```python
from build123d import *

# Parameters (mm, degrees)
SKETCH_1_W                         = 54
SKETCH_1_H                         = 25
SKETCH_1_R                         = 4
SKETCH_1_R_2                       = 1.5
SM_BASE_FLANGE_1_DEPTH             = 2
SM_EDGE_FLANGE_1_STRIP_W           = 10.4732
SM_EDGE_FLANGE_1_STRIP_H           = 2
SM_EDGE_FLANGE_1_STRIP_CUT_DEPTH   = 25
SM_EDGE_FLANGE_1_STRIP_2_W         = 10.4732
SM_EDGE_FLANGE_1_STRIP_2_H         = 2
SM_EDGE_FLANGE_1_STRIP_CUT_2_DEPTH = 25
SM_EDGE_FLANGE_1_DEPTH             = 25
SM_EDGE_FLANGE_1_BEND_DEPTH        = 25
SKETCH_12_R                        = 4
SKETCH_12_R_2                      = 1.5
CUT_EXTRUDE_1_DEPTH                = 72


# Sheet-metal steps are written as plain solids
with BuildPart() as part:
    # Sketch 1 → 基体-法兰1 (new body)
    with BuildSketch(Plane.XY):
        with Locations((27, -12.5)):
            Rectangle(SKETCH_1_W, SKETCH_1_H)
        with Locations((27, -12.5)):
            Circle(SKETCH_1_R, mode=Mode.SUBTRACT)
        with Locations((27, -5.5)):
            Circle(SKETCH_1_R_2, mode=Mode.SUBTRACT)
        with Locations((27, -19.5)):
            Circle(SKETCH_1_R_2, mode=Mode.SUBTRACT)
        with Locations((34, -12.5)):
            Circle(SKETCH_1_R_2, mode=Mode.SUBTRACT)
        with Locations((20, -12.5)):
            Circle(SKETCH_1_R_2, mode=Mode.SUBTRACT)
        with Locations((45.5, -12.5)):
            Circle(SKETCH_1_R_2, mode=Mode.SUBTRACT)
        with Locations((8.5, -12.5)):
            Circle(SKETCH_1_R_2, mode=Mode.SUBTRACT)
    extrude(amount=-SM_BASE_FLANGE_1_DEPTH)

    # 边线-法兰1 strip (across the edge) → 边线-法兰1 strip cut (cut)
    with BuildSketch(Plane(origin=(-1, 0, 0), x_dir=(1, 0, 0), z_dir=(0, -1, 0))):
        with Locations((-2.5, -1)):
            Rectangle(SM_EDGE_FLANGE_1_STRIP_W, SM_EDGE_FLANGE_1_STRIP_H)
    extrude(amount=SM_EDGE_FLANGE_1_STRIP_CUT_DEPTH, mode=Mode.SUBTRACT)

    # 边线-法兰1 strip 2 (across the edge) → 边线-法兰1 strip cut 2 (cut)
    with BuildSketch(Plane(origin=(55, -25, 0), x_dir=(-1, 0, 0), z_dir=(0, 1, 0))):
        with Locations((-2.5, -1)):
            Rectangle(SM_EDGE_FLANGE_1_STRIP_2_W, SM_EDGE_FLANGE_1_STRIP_2_H)
    extrude(amount=SM_EDGE_FLANGE_1_STRIP_CUT_2_DEPTH, mode=Mode.SUBTRACT)

    # 边线-法兰1 section (across the edge) → 边线-法兰1 (add)
    with BuildSketch(Plane(origin=(-1, 0, 0), x_dir=(1, 0, 0), z_dir=(0, -1, 0))):
        with BuildLine():
            Line((0, 0.7366), (0, 68))
            Line((0, 68), (2, 68))
            Line((2, 68), (2, 0.7366))
            ThreePointArc((2, 0.7366), (2.215745145, 0.215745145), (2.7366, 0))
            Line((2.7366, 0), (2.7366, -2))
            ThreePointArc((2.7366, -2), (0.801531583, -1.198468417), (0, 0.7366))
        make_face()
    extrude(amount=SM_EDGE_FLANGE_1_DEPTH)

    # 边线-法兰1 section 2 (across the edge) → 边线-法兰1 bend (add)
    with BuildSketch(Plane(origin=(55, -25, 0), x_dir=(-1, 0, 0), z_dir=(0, 1, 0))):
        with BuildLine():
            Line((0, 0.7366), (0, 68))
            Line((0, 68), (2, 68))
            Line((2, 68), (2, 0.7366))
            ThreePointArc((2, 0.7366), (2.215745145, 0.215745145), (2.7366, 0))
            Line((2.7366, 0), (2.7366, -2))
            ThreePointArc((2.7366, -2), (0.801531583, -1.198468417), (0, 0.7366))
        make_face()
    extrude(amount=SM_EDGE_FLANGE_1_BEND_DEPTH)

    # 草图12 → 切除-拉伸1 (cut)
    with BuildSketch(Plane(origin=(55, 0, 0), x_dir=(0, 0, -1), z_dir=(1, 0, 0))):
        with Locations(Location((-50, -12.5, 0), (0, 0, 180))):
            Circle(SKETCH_12_R)
        with Locations(Location((-57, -12.5, 0), (0, 0, 180))):
            Circle(SKETCH_12_R_2)
        with Locations(Location((-50, -5.5, 0), (0, 0, 180))):
            Circle(SKETCH_12_R_2)
        with Locations(Location((-43, -12.5, 0), (0, 0, 180))):
            Circle(SKETCH_12_R_2)
        with Locations(Location((-50, -19.5, 0), (0, 0, 180))):
            Circle(SKETCH_12_R_2)
        with Locations(Location((-31.5, -12.5, 0), (0, 0, 180))):
            Circle(SKETCH_12_R_2)
        with Locations(Location((-14.5, -12.5, 0), (0, 0, 180))):
            Circle(SKETCH_12_R_2)
        with BuildLine():
            Line((-49.5, -25), (-68, -25))
            Line((-68, -25), (-68, 0))
            Line((-68, 0), (-49.5, 0))
            ThreePointArc((-49.5, 0), (-62, -12.5), (-49.5, -25))
        make_face()
    extrude(amount=-CUT_EXTRUDE_1_DEPTH, mode=Mode.SUBTRACT)


solid = part.part
```
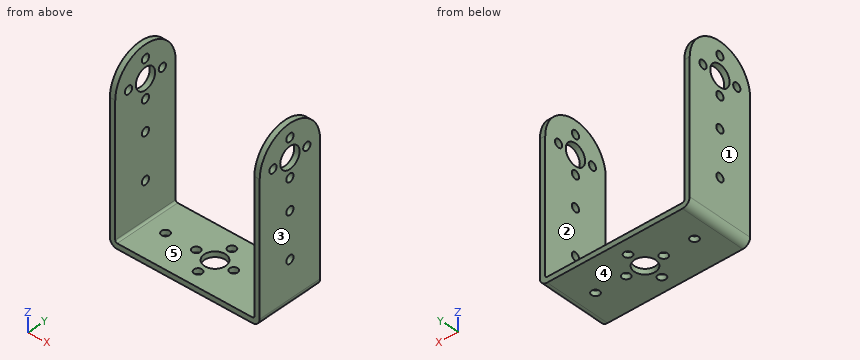
Design review of the part built by this model. Coordinates are the model's own, in mm. Face numbers are marked on the shaded views. A direction names the side the tool comes from. Coordinates: 2 decimals unless noted, no trailing zeros. Order: outer loops, then holes, each group sorted by start corner. A loop starts at its lowest first (then second) coordinate and runs counter-clockwise, first axis right, second up. Notation, with made-up numbers: (32.25, 26.5) - (84.25, 26.5) arc R13 cw to (84.25, 42.5) - close; hole circle Ø6 at (39, 67.5). An arc over 180 degrees is marked (long way). Answer in a Markdown table with one row per item.
(1) Wall thickness on line 1 along X through (y, z) = (-3.5, 3); line 2 along Y through (x, z) = (-0.2, 43); line 3 along Z through (x, y) = (0.2, -12.5): over which ranges is each line inside the solid? List them lowest first. Write a range as from..to.
Checked values:
| item | result |
|---|---|
| line 1 | -1..1, 53..55 |
| line 2 | -25..-14, -11..0 |
| line 3 | -1.53..13, 16..30, 33..41.5, 44.5..46, 54..55.5, 58.5..62 |
(2) Consider section B-B on x = 20. State the section outline as (y, z) points, plus the area to 3 significant figures.
Checked values:
| item | result |
|---|---|
| outline | (-25, -2) - (-14, -2) - (-14, 0) - (-25, 0) - close; (-11, -2) - (0, -2) - (0, 0) - (-11, 0) - close |
| area | 44.0 mm^2 |
(3) Clearance check with a flat-ended pin moving along its axis: pin 1 (2 mm diameter, centred on x = 13.5, y = -19, fed in from +Z). State where the tip first meets the part, or that it passes through.
Checked values:
| item | result |
|---|---|
| pin 1 | z = 0 |
(4) Consider section D-D on z = 52.5. State the section outline as (x, y) points.
Checked values:
| item | result |
|---|---|
| outline | (-1, -24.63) - (1, -24.63) - (1, -15.62) - (-1, -15.62) - close; (-1, -9.38) - (1, -9.38) - (1, -0.37) - (-1, -0.37) - close; (53, -24.63) - (55, -24.63) - (55, -15.62) - (53, -15.62) - close; (53, -9.38) - (55, -9.38) - (55, -0.37) - (53, -0.37) - close |
(5) Consider section A-A on z = 11.5. State the section outline as (x, y) points.
Checked values:
| item | result |
|---|---|
| outline | (-1, -25) - (1, -25) - (1, 0) - (-1, 0) - close; (53, -25) - (55, -25) - (55, 0) - (53, 0) - close |
(6) For the marked faces 4 and 5, list the 3-axis set-ups (+Z, -Z, +X, -X, +Y, -Y) from which the entire face can be reached by the end or side of a thin tool; tool diameter is ignored.
Checked values:
| item | result |
|---|---|
| face 4 | -Z, +X, -X, +Y, -Y |
| face 5 | +Z, +Y, -Y |
(7) Consider section C-C on y = -4.75. State the section outline as (x, z) points, plus the area to 3 significant figures.
Checked values:
| item | result |
|---|---|
| outline | (-1, 0.74) arc R2.74 ccw to (1.74, -2) - (25.7, -2) - (25.7, 0) - (1.74, 0) arc R0.74 cw to (1, 0.74) - (1, 48.7) - (-1, 48.7) - close; (-1, 51.3) - (1, 51.3) - (1, 59.31) - (-1, 59.31) - close; (28.3, -2) - (52.26, -2) arc R2.74 ccw to (55, 0.74) - (55, 48.7) - (53, 48.7) - (53, 0.74) arc R0.74 cw to (52.26, 0) - (28.3, 0) - close; (53, 51.3) - (55, 51.3) - (55, 59.31) - (53, 59.31) - close |
| area | 331 mm^2 |
(8) The part is to be moulded in two halves that separate along X. For the marked faces 1, 2 and 3, say which applies: released by +X, released by -X, zero draft, split by the parting line, or undercut.
Checked values:
| item | result |
|---|---|
| face 1 | released by -X |
| face 2 | undercut |
| face 3 | released by +X |
